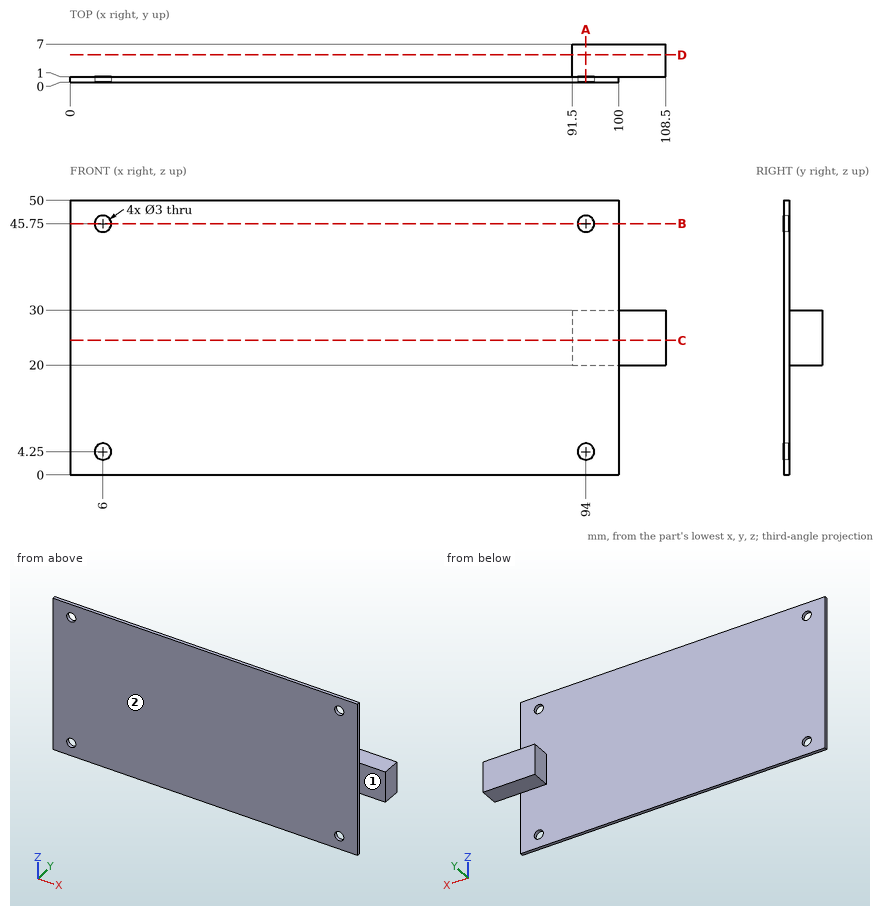
Part print with two shaded views. Sizes in mm from the minimum x, y, z corner. A direction names the side the tool comes from. Coordinates: 2 decimals unless noted, no trailing zeros. Order: outer loops, then holes, each group sorted by start corner. A loop starts at its lowest first (then second) coordinate and runs counter-clockwise, first axis right, second up. Notation, with made-up numbers: M 66,80.5 L 81,80.5 A6 cw 81,89.5 Z; hole C -36.5,-3 d7. An arc over 180 degrees is marked long. Use a Markdown table: item, result.
(1) Cut at B-B on z = 45.75. Write the cut outline in (x, y), then the cut area to 3 significant figures.
A:
| item | result |
|---|---|
| outline | M 0,0 L 4.5,0 L 4.5,1 L 0,1 Z; M 7.5,0 L 92.5,0 L 92.5,1 L 7.5,1 Z; M 95.5,0 L 100,0 L 100,1 L 95.5,1 Z |
| area | 94.0 mm^2 |
(2) Cut at C-C on z = 24.5. Write the cut outline in (x, y), then the cut area to 3 significant figures.
A:
| item | result |
|---|---|
| outline | M 0,0 L 100,0 L 100,1 L 108.5,1 L 108.5,7 L 91.5,7 L 91.5,1 L 0,1 Z |
| area | 202 mm^2 |
(3) Tool access for the marked faces 1 and 2: list every direction of +Z, -Z, +X, -X, +Y, -Y with a clear straight run to the whole face (end or side of a thin tool).
A:
| item | result |
|---|---|
| face 1 | +Z, -Z, +X, -Y |
| face 2 | +Z, -Z, +X, -X, -Y |
(4) Cut at A-A on x = 94. Write the cut outline in (y, z).
A:
| item | result |
|---|---|
| outline | M 0,0 L 1,0 L 1,2.75 L 0,2.75 Z; M 0,5.75 L 1,5.75 L 1,20 L 7,20 L 7,30 L 1,30 L 1,44.25 L 0,44.25 Z; M 0,47.25 L 1,47.25 L 1,50 L 0,50 Z |
(5) Cut at D-D on y = 5. Write the cut outline in (x, z).
A:
| item | result |
|---|---|
| outline | M 91.5,20 L 108.5,20 L 108.5,30 L 91.5,30 Z |
(6) Flat gauge pins, fed straight in: pin 1 (15 mm diameter, centred on x = 67.5, z = 34, fed in from +Y); pin 2 (3 mm diameter, centred on y = 2, z = 30, fed in from -X); pin 3 (2.5 mm diameter, centred on x = 6, z = 45.75, fed in from -Y); pin 4 (1.5 mm diameter, centred on y = 1, z = 8, fed in from +X). Where does each tip first touch, or does it go through?
A:
| item | result |
|---|---|
| pin 1 | stops at y = 1 |
| pin 2 | stops at x = 0 |
| pin 3 | passes through |
| pin 4 | stops at x = 100 |
(7) Probe L1, parallel to X at y = 0.85, z = 45.75; L2, parallel to Z at x = 94, y = 0.25; L3, parallel to Y at x = 27.5, z = 13.5. List the from-to ranges inside material, lowest first.
A:
| item | result |
|---|---|
| L1 | x = 0 to 4.5, 7.5 to 92.5, 95.5 to 100 |
| L2 | z = 0 to 2.75, 5.75 to 44.25, 47.25 to 50 |
| L3 | y = 0 to 1 |
